Autodesk Inventor part; units mm, degrees
ref_plane "YZ Plane" through (0, 0, 0) normal (1, 0, 0) x (0, 1, 0)
ref_plane "XZ Plane" through (0, 0, 0) normal (0, 1, 0) x (-1, 0, 0)
ref_plane "XY Plane" through (0, 0, 0) normal (0, 0, 1) x (1, 0, 0)
sketch "스케치1" plane through (0, 0, 0) normal (0, 0, 1) x (1, 0, 0)
  line L0 (-32.5, 45) -> (32.5, 45)
  line L1 (32.5, 45) -> (32.5, -45)
  line L2 (32.5, -45) -> (-32.5, -45)
  line L3 (-32.5, -45) -> (-32.5, 45)
  line L4 (-32.5, 45) -> (32.5, -45) construction
  line L5 (32.5, 45) -> (-32.5, -45) construction
  point P0 (0, 0)
  dimension "d1" = 65
  dimension "d2" = 90
extrude "돌출1" add sketch "스케치1" along normal blind 2
sketch "스케치2" plane through (0, 0, 2) normal (0, 0, 1) x (1, 0, 0)
  circle A0 centre (-24, -31) radius 2
  line L0 (-32.5, -45) -> (32.5, -45)
  line L1 (-32.5, 45) -> (-32.5, -45)
  circle A1 centre (24, -31) radius 2
  line L2 (32.5, -45) -> (32.5, 45)
  circle A2 centre (-19, 20.5) radius 2
  circle A3 centre (9, 20.5) radius 2
  point P0 (0, 0)
  dimension "d14" = 4
  dimension "d15" = 14
  dimension "d16" = 8.5
  dimension "d17" = 4
  dimension "d18" = 14
  dimension "d19" = 8.5
  dimension "d20" = 4
  dimension "d21" = 65.5
  dimension "d22" = 13.5
  dimension "d23" = 4
  dimension "d24" = 23.5
  dimension "d25" = 65.5
extrude "돌출2" cut sketch "스케치2" against normal blind 2
sketch "스케치3" plane through (0, 0, 2) normal (0, 0, 1) x (1, 0, 0)
  line L0 (32.5, -45) -> (32.5, 45)
  line L1 (-32.5, -45) -> (32.5, -45)
  line L2 (32.5, -45) -> (32.5, 45)
  line L3 (32.5, 45) -> (-32.5, 45)
  line L4 (-32.5, 45) -> (-32.5, -45)
  line L5 (-32.5, -45) -> (32.5, 45) construction
  line L6 (32.5, -45) -> (-32.5, 45) construction
  line L7 (-31.5, -44) -> (31.5, -44)
  line L8 (31.5, -44) -> (31.5, 44)
  line L9 (31.5, 44) -> (-31.5, 44)
  line L10 (-31.5, 44) -> (-31.5, -44)
  line L11 (-31.5, -44) -> (31.5, 44) construction
  line L12 (31.5, -44) -> (-31.5, 44) construction
  point P0 (0, 0)
  dimension "d28" = 63
  dimension "d29" = 88
extrude "돌출3" add sketch "스케치3" along normal blind 20
properties part number "case"
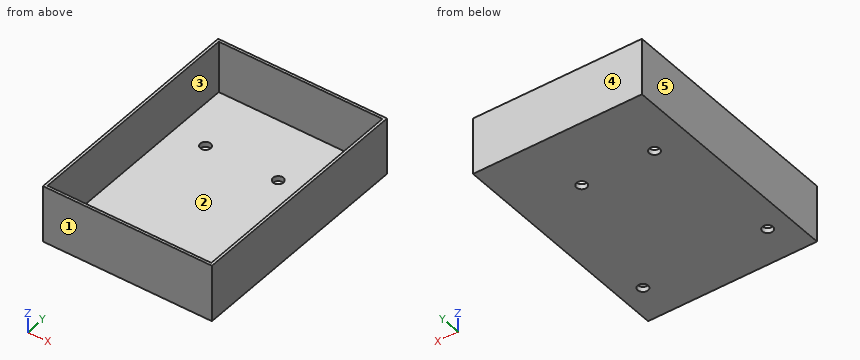
For this review, take the finished solid that the model builds, in its own axes (mm). Face numbers are marked on the shaded views. A direction names the side the tool comes from. Coordinates: 2 decimals unless noted, no trailing zeros. Loops run counter-clockwise (first coordinate to the right, second up) from the corner with the lowest first, then second, coordinate; pieces in that order, holes last. Notation, with made-up numbers: (33.25, -15.75) - (74.25, -15.75) arc R32 ccw to (74.25, 13.25) - close; hole circle Ø5 at (36, -19.75). An arc over 180 degrees is marked (long way). Return JSON: item names as keys, results as strings.
Item 1: Take a section at D-D (x = -10). Give the boundary of the cut face in (y, z).
Determined:
{"outline": "(-45, 0) - (45, 0) - (45, 22) - (44, 22) - (44, 2) - (-44, 2) - (-44, 22) - (-45, 22) - close"}
Item 2: For the marked faces 1 and 2, list the 3-axis set-ups (+Z, -Z, +X, -X, +Y, -Y) from which the entire face can be reached by the end or side of a thin tool; tool diameter is ignored.
Determined:
{"face 1": "+Z, -Z, +X, -X, -Y", "face 2": "+Z"}
Item 3: Mouldability with a two-part tool opening along X and no side actions: class the marked faces 3, 4 and 5 as pulls with the +X half, pulls with the -X half, needs draft (parallel to the pull), parting line crosses it, or undercut.
Determined:
{"face 3": "undercut", "face 4": "needs draft", "face 5": "pulls with the -X half"}
Item 4: Take a section at B-B (y = 12.5). Give the boundary of the cut face in (x, z), then the cut area to 3 significant figures.
Determined:
{"outline": "(-32.5, 0) - (32.5, 0) - (32.5, 22) - (31.5, 22) - (31.5, 2) - (-31.5, 2) - (-31.5, 22) - (-32.5, 22) - close", "area": "170 mm2"}
Item 5: Take a section at A-A (x = -24). Give the boundary of the cut face in (y, z).
Determined:
{"outline": "(-45, 0) - (-33, 0) - (-33, 2) - (-44, 2) - (-44, 22) - (-45, 22) - close; (-29, 0) - (45, 0) - (45, 22) - (44, 22) - (44, 2) - (-29, 2) - close"}
Item 6: Take a section at C-C (z = 14). Give the boundary of the cut face in (x, y).
Determined:
{"outline": "(-32.5, -45) - (32.5, -45) - (32.5, 45) - (-32.5, 45) - close; hole (-31.5, -44) - (31.5, -44) - (31.5, 44) - (-31.5, 44) - close"}
Item 7: Insertion check: pin 1 (4 mm diameter, centred on x = -18.5, y = -31, fed in from +Z); pin 2 (6.5 mm diameter, centred on x = -24, y = -31, fed in from -Z). Each pin has a flat end and moves straight along its axis. Give the tip position at first contact, or say it passes through.
Determined:
{"pin 1": "stops at z = 2", "pin 2": "stops at z = 0"}
Item 8: For line 1 (Y direction, x = -24, z = 7); line 2 (Y direction, x = 24, z = 0.55); line 3 (X direction, y = 31.5, z = 15.5), list the stretches that pass through material, from the lowest coordinate up.
Determined:
{"line 1": "y = -45 to -44, 44 to 45", "line 2": "y = -45 to -33, -29 to 45", "line 3": "x = -32.5 to -31.5, 31.5 to 32.5"}
